from build123d import *

# Parameters (mm, degrees)
F0_W      = 139.7
F0_H      = 127
F1_DEPTH  = 139.7
F2_W      = 137.16
F2_H      = 137.16
F3_DEPTH  = 124.46
F5_DEPTH  = 25.4
F7_DEPTH  = 25.4
F9_DEPTH  = 25.4
F11_DEPTH = 25.4
F12_R     = 50.8
F14_DEPTH = 2.54


with BuildPart() as f1:
    # F0 (on Top) → F1 (new body)
    with BuildSketch(Plane.XY):
        with Locations((-69.85, -63.5)):
            Rectangle(F0_W, F0_H)
    extrude(amount=F1_DEPTH)

    # F2 (on face) → F3 (cut)
    with BuildSketch(Plane.XZ.offset(127)):
        with Locations((-68.58, 71.12)):
            Rectangle(F2_W, F2_H)
    extrude(amount=-F3_DEPTH, mode=Mode.SUBTRACT)

    # F4 (on face) → F5 (cut)
    with BuildSketch(Plane.XZ.offset(2.54)):
        Polygon((-6.9185560569, 178.2889813185), (-137.16, 139.7), (0, 2.54), (55.8031983674, 142.7505463362), align=None)
    extrude(amount=-F5_DEPTH, mode=Mode.SUBTRACT)

    # F6 (on face) → F7 (cut)
    with BuildSketch(Plane.XZ.offset(2.54)):
        Polygon((-137.16, 104.14), (-137.16, 2.54), (-35.56, 2.54), align=None)
    extrude(amount=-F7_DEPTH, mode=Mode.SUBTRACT)

    # F8 (on face) → F9 (cut)
    with BuildSketch(Plane.XY.offset(2.54)):
        with BuildLine():
            Line((-137.16, -38.1), (-137.16, -88.9))
            Line((-137.16, -88.9), (-48.26, -88.9))
            ThreePointArc((-48.26, -88.9), (-22.86, -63.5), (-48.26, -38.1))
            Line((-48.26, -38.1), (-137.16, -38.1))
        make_face()
    extrude(amount=-F9_DEPTH, mode=Mode.SUBTRACT)

    # F10 (on face) → F11 (cut)
    with BuildSketch(Plane.YZ.offset(-137.16)):
        with BuildLine():
            Line((-38.1, 0), (-38.1, 2.54))
            Line((-38.1, 2.54), (-38.1, 91.44))
            ThreePointArc((-38.1, 91.44), (-63.5, 116.84), (-88.9, 91.44))
            Line((-88.9, 91.44), (-88.9, 2.54))
            Line((-88.9, 2.54), (-88.9, 0))
            Line((-88.9, 0), (-38.1, 0))
        make_face()
    extrude(amount=-F11_DEPTH, mode=Mode.SUBTRACT)

    # F12
    f12_edges = [f1.edges().sort_by_distance(p)[0] for p in [
        (0, -127, 1.27),
        (-138.43, -127, 139.7),
    ]]
    fillet(f12_edges, radius=F12_R)

    # F13 (on face) → F14 (join)
    with BuildSketch(Plane(origin=(-139.7, 0, 0), x_dir=(0, -1, 0), z_dir=(-1, 0, 0))):
        Polygon((38.1, 74.93), (38.1, 69.85), (38.1, 64.77), (88.9, 64.77), (88.9, 69.85), (88.9, 74.93), align=None)
    extrude(amount=-F14_DEPTH)


solid = f1.part
CAD build for the part. Positions are in the model's coordinates, mm. A direction names the side the tool comes from. Round coordinates to 2 decimals unless told otherwise and drop trailing zeros. Order: outer loops, then holes, each group sorted by start corner. A loop starts at its lowest first (then second) coordinate and runs counter-clockwise, first axis right, second up. Notation, with made-up numbers: (-6.5, 8) - (0.5, 8) arc R30 cw to (0.5, 40) - close; hole circle Ø11 at (73, 55.25). An arc over 180 degrees is marked (long way). Return JSON: item names as keys, results as strings.
(1) Pin check, flat tips, straight feed: pin 1 Ø1.3 at (x, z) = (-138, 82.5) entering from +Y; pin 2 Ø1.3 at (x, y) = (-138, -54) entering from -Z; pin 3 Ø2 at (y, z) = (-110, 122) entering from +X; pin 4 Ø1 at (x, z) = (-32.5, 35.5) entering from -Y. Stop position of each tip, or through.
Answer key:
{"pin 1": "stops at y = 0", "pin 2": "stops at z = 64.77", "pin 3": "stops at x = -137.16", "pin 4": "stops at y = -2.54"}
(2) Cut at D-D (x = -31.5). Give the cut face in (y, z).
Answer key:
{"outline": "(-123.19, 0) - (-82.59, 0) - (-82.59, 2.54) - (-123.19, 2.54) - close; (-44.41, 0) - (0, 0) - (0, 34.04) - (-2.54, 34.04) - (-2.54, 2.54) - (-44.41, 2.54) - close"}
(3) Cut at A-A (z = 34). Give the cut face in (x, y), then the cut area to 3 significant figures.
Answer key:
{"outline": "(-139.7, -127) - (-137.16, -127) - (-137.16, -88.9) - (-139.7, -88.9) - close; (-139.7, -38.1) - (-137.16, -38.1) - (-137.16, 0) - (-139.7, 0) - close; (-67.02, -2.54) - (-31.46, -2.54) - (-31.46, 0) - (-67.02, 0) - close", "area": "284 mm^2"}
(4) Wall check: probe 1 along Y at (x, z) = (-47.5, 21); probe 2 along Z at (x, y) = (-129, -7.5); probe 3 along X at (y, z) = (-115.5, 117.5). Give the ranges that are in metal, low to high. Write a range as from..to.
Answer key:
{"probe 1": "y = -2.54..0", "probe 2": "z = 0..2.54", "probe 3": "x = -139.7..-137.16"}
(5) Cut at C-C (y = -26). Give the cut face in (x, z).
Answer key:
{"outline": "(-139.7, 0) - (0, 0) - (0, 2.54) - (-137.16, 2.54) - (-137.16, 139.7) - (-139.7, 139.7) - close"}
(6) Tool access for faces 1 (the face through (-114, -88.9, 1)), 2 (the face through (-79, -2.54, 66)), 3 (the face through (-22.866, -64.059, 1.288)): list every direction of +Z, -Z, +X, -X, +Y, -Y with a clear straight run to the whole face (end or side of a thin tool).
Answer key:
{"face 1": "-Z, -X", "face 2": "+Z, +X, -Y", "face 3": "+Z, -Z, -X"}
(7) Pull direction Z, two halves, no side cores. Call faces 4 (the face through (-69.54, -1.29, 72.08)), 5 (the face through (-138.412, -62.941, 116.834)), 6 (the face through (-114, -38.1, 1)), 7 (the face through (-85.65, -1.29, 52.63)): +Z half, -Z half, draft (parallel to the pull), parting line (faces both ways), or undercut.
Answer key:
{"face 4": "+Z half", "face 5": "undercut", "face 6": "draft", "face 7": "undercut"}
(8) Cut at B-B (x = -103). Give the cut face in (y, z), then the cut area to 3 significant figures.
Answer key:
{"outline": "(-127, 0) - (-88.9, 0) - (-88.9, 2.54) - (-127, 2.54) - close; (-38.1, 0) - (0, 0) - (0, 2.54) - (-38.1, 2.54) - close; (-2.54, 69.98) - (0, 69.98) - (0, 105.54) - (-2.54, 105.54) - close", "area": "284 mm^2"}
